Source: CAD feature listing. Evaluate the final solid. Frame: model axes, mm. Face numbers are marked on the shaded views. A direction names the side the tool comes from. Coordinates: 2 decimals unless noted, no trailing zeros. Order: outer loops, then holes, each group sorted by start corner. A loop starts at its lowest first (then second) coordinate and runs counter-clockwise, first axis right, second up.
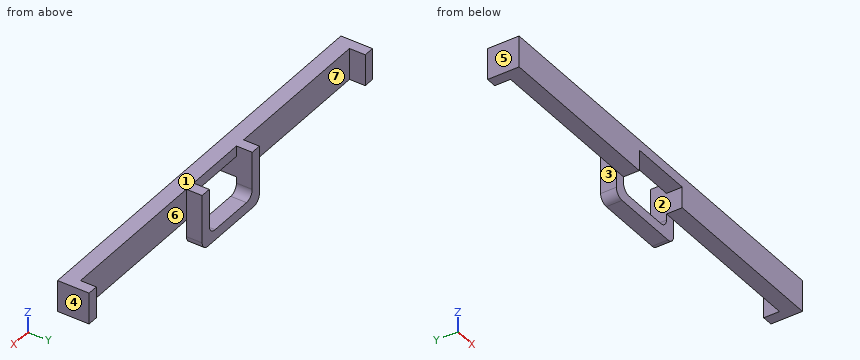
```python
from build123d import *

# Parameters (mm, degrees)
EXTRUDE_1_DEPTH          = 15
EXTRUDE_2_DEPTH          = 15
CUT_EXTRUDE_1_DEPTH      = 101.410407827
CUT_EXTRUDE_1_DEPTH_BACK = 101.410407827
SKETCH_3_W               = 30
SKETCH_3_H               = 10
EXTRUDE_3_DEPTH          = 7.5


with BuildPart() as part:
    # 草图1 → 凸台-拉伸1 (new body)
    with BuildSketch(Plane.XY):
        Polygon((-94, 7.5), (-99, 7.5), (-99, -7.5), (99, -7.5), (99, 7.5), (94, 7.5), (94, 0), (-94, 0), align=None)
    extrude(amount=EXTRUDE_1_DEPTH)

    # 草图2 → 凸台-拉伸2 (add)
    with BuildSketch(Plane.XY.offset(15)):
        Polygon((20, -7.5), (-20, -7.5), (-20, 7.5), (-15, 7.5), (-15, 0), (15, 0), (15, 7.5), (20, 7.5), align=None)
    extrude(amount=-EXTRUDE_2_DEPTH)

    # 草图3 → 切除-拉伸1 (cut, two sides: drawn at the far end of the back side and taken through both)
    with BuildSketch(Plane(origin=(0, 0, 0), x_dir=(1, 0, 0), z_dir=(0, 1, 0)).offset(-CUT_EXTRUDE_1_DEPTH_BACK)):
        with Locations((0, -5)):
            Rectangle(SKETCH_3_W, SKETCH_3_H)
    extrude(amount=CUT_EXTRUDE_1_DEPTH + CUT_EXTRUDE_1_DEPTH_BACK, mode=Mode.SUBTRACT)

    # 草图4 → 凸台-拉伸3 (add)
    with BuildSketch(Plane(origin=(0, 0, 0), x_dir=(1, 0, 0), z_dir=(0, 1, 0))):
        with BuildLine():
            Line((-15, -11.176683095), (-15, 3))
            ThreePointArc((-15, 3), (-13.828427125, 5.828427125), (-11, 7))
            Line((-11, 7), (11, 7))
            ThreePointArc((11, 7), (13.828427125, 5.828427125), (15, 3))
            Line((15, 3), (15, 0))
            Line((15, 0), (20, 0))
            Line((20, 0), (20, 8))
            ThreePointArc((20, 8), (18.828427125, 10.828427125), (16, 12))
            Line((16, 12), (-16, 12))
            ThreePointArc((-16, 12), (-18.828427125, 10.828427125), (-20, 8))
            Line((-20, 8), (-20, -11.176683095))
            Line((-20, -11.176683095), (-15, -11.176683095))
        make_face()
    extrude(amount=EXTRUDE_3_DEPTH)


solid = part.part
```
Q1. Section query D-D on z = 12.5. Output: boundary loops of the cut face in (x, y), plus the area to 4 significant figures.
Solutions:
outline: (-99, -7.5) - (99, -7.5) - (99, 7.5) - (94, 7.5) - (94, 0) - (20, 0) - (20, 7.5) - (15, 7.5) - (15, 0) - (-15, 0) - (-15, 7.5) - (-20, 7.5) - (-20, 0) - (-94, 0) - (-94, 7.5) - (-99, 7.5) - close
area: 1,635 mm2
Q2. Pull-direction query (X, two-part tool) for the marked faces 4, 5, 6 and 7; classes: pulls with the +X half, pulls with the -X half, needs draft (parallel to the pull), parting line crosses it, or undercut.
Solutions:
face 4: pulls with the +X half
face 5: pulls with the -X half
face 6: undercut
face 7: undercut
Q3. Section query C-C on x = 8. Output: boundary loops of the cut face in (y, z), plus the area to 3 significant figures.
Solutions:
outline: (-7.5, 10) - (0, 10) - (0, 15) - (-7.5, 15) - close; (0, -12) - (7.5, -12) - (7.5, -7) - (0, -7) - close
area: 75.0 mm2
Q4. Material intervals for line 1 along X through (y, z) = (3.5, 1.75); line 2 along X through (y, z) = (-1.5, 1); line 3 along Z through (x, y) = (2, -5.5), sorted ascending.
Solutions:
line 1: x = -99 to -94, -20 to -15, 15 to 20, 94 to 99
line 2: x = -99 to -15, 15 to 99
line 3: z = 10 to 15
Q5. Set-up query: the marked faces 1, 2 and 3. Return all of +Z, -Z, +X, -X, +Y, -Y with unobstructed straight access to the full face (end or side cutting, diameter ignored); none if empty.
Solutions:
face 1: +Z, +X, -X, +Y, -Y
face 2: +Y
face 3: +Z, -Z, +Y
Q6. Section query B-B on y = 4. Output: boundary loops of the cut face in (x, z).
Solutions:
outline: (-99, 0) - (-94, 0) - (-94, 15) - (-99, 15) - close; (-20, -8) arc R4 ccw to (-16, -12) - (16, -12) arc R4 ccw to (20, -8) - (20, 15) - (15, 15) - (15, -3) arc R4 cw to (11, -7) - (-11, -7) arc R4 cw to (-15, -3) - (-15, 15) - (-20, 15) - close; (94, 0) - (99, 0) - (99, 15) - (94, 15) - close
Q7. Section query A-A on z = 3. Output: boundary loops of the cut face in (x, y).
Solutions:
outline: (-99, -7.5) - (-15, -7.5) - (-15, 7.5) - (-20, 7.5) - (-20, 0) - (-94, 0) - (-94, 7.5) - (-99, 7.5) - close; (15, -7.5) - (99, -7.5) - (99, 7.5) - (94, 7.5) - (94, 0) - (20, 0) - (20, 7.5) - (15, 7.5) - close
Q8. Pin query (flat end, axial travel): P1, Ø8, axis at x = -5.5, y = -5.5, coming from the -Z side; P2, Ø2, axis at x = -1.5, y = 3.5, coming from the +Z side; P3, Ø1.5, axis at x = 5, z = 13, coming from the +Y side; P4, Ø4.5, axis at x = -70, y = 2.5, coming from the -Z side. Return the tip coordinate at first contact, or that it passes through.
Solutions:
P1: stops at z = 10
P2: stops at z = -7
P3: stops at y = 0
P4: passes through
